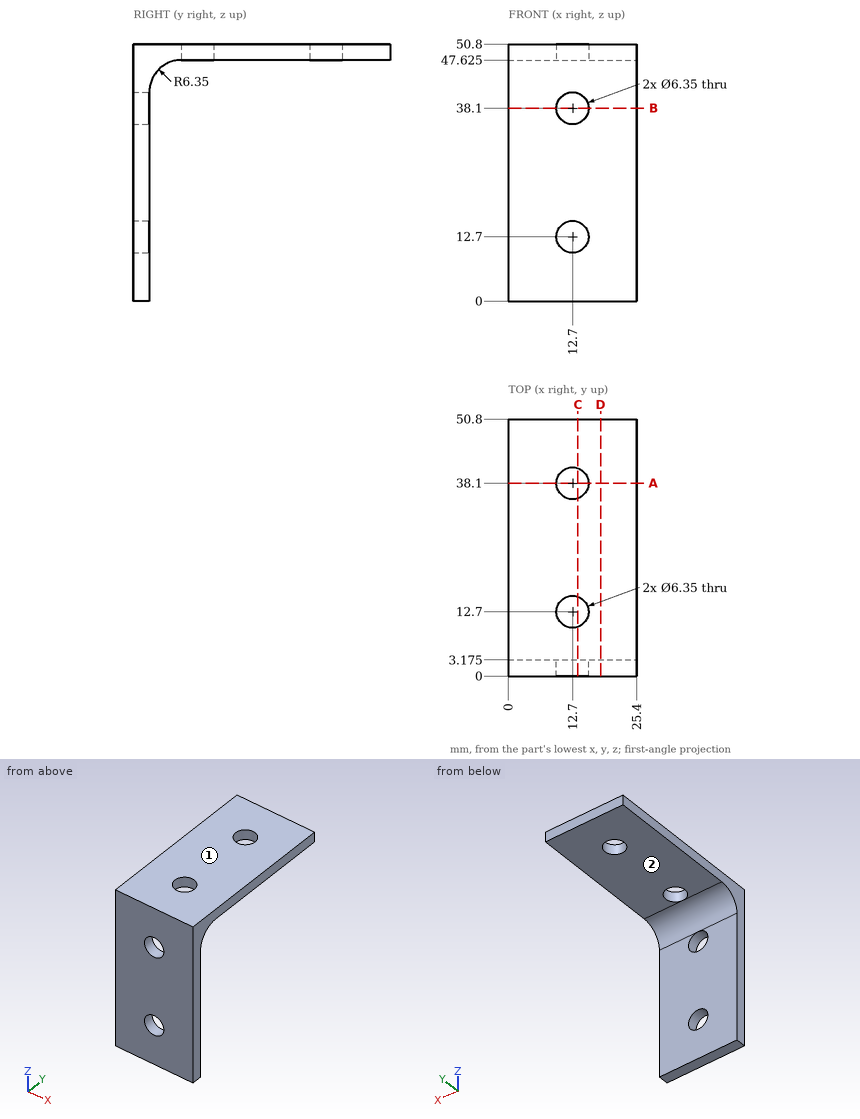
Study the drawing (mm; zero at the part's minimum x, y, z) and answer. A direction names the side the tool comes from. Give positions to 0.01 mm unless a question says otherwise; leave off trailing zeros. Order: outer loops, then holes, each group sorted by start corner. A loop starts at its lowest first (then second) coordinate and runs counter-clockwise, first axis right, second up.
1. Section A-A, the plane y = 38.1 is taken. Determine the outline of the cut face in (x, z) (3 decimals), and give its area (3 significant figures).
Result sheet:
outline: (0, 47.625) - (9.525, 47.625) - (9.525, 50.8) - (0, 50.8) - close; (15.875, 47.625) - (25.4, 47.625) - (25.4, 50.8) - (15.875, 50.8) - close
area: 60.5 mm2
2. For the marked faces 1 and 2, determine the directions among +Z, -Z, +X, -X, +Y, -Y from which every point of the face is accessible in a straight line to the end or side of a thin tool.
Result sheet:
face 1: +Z, +X, -X, +Y, -Y
face 2: -Z, +X, -X, +Y
3. Straight lines are drawn through the part: L1, parallel to Z at x = 12.7, y = 0.8 (3 decimals); L2, parallel to X at y = 38, z = 49. For each, find the intervals that lie inside material, in ascending order.
Result sheet:
L1: z = 0 to 9.525, 15.875 to 34.925, 41.275 to 50.8
L2: x = 0 to 9.53, 15.87 to 25.4
4. Section C-C, the plane x = 13.75 is taken. Determine the outline of the cut face in (y, z) (3 decimals), and give its area (3 significant figures).
Result sheet:
outline: (0, 0) - (3.175, 0) - (3.175, 9.704) - (0, 9.704) - close; (0, 15.696) - (3.175, 15.696) - (3.175, 35.104) - (0, 35.104) - close; (0, 41.096) - (3.175, 41.096) - (3.175, 41.275) arc R6.35 cw to (9.525, 47.625) - (9.704, 47.625) - (9.704, 50.8) - (0, 50.8) - close; (15.696, 47.625) - (35.104, 47.625) - (35.104, 50.8) - (15.696, 50.8) - close; (41.096, 47.625) - (50.8, 47.625) - (50.8, 50.8) - (41.096, 50.8) - close
area: 245 mm2
5. Each of these flat-tipped pins is pushed along its axis until it touches: P1, Ø8, axis at x = 22, y = 12, coming from the -Z side; P2, Ø4, axis at x = 12.7, y = 38.1, coming from the -Z side; P3, Ø1, axis at x = 15.5, z = 26.5, coming from the +Y side (3 decimals). Where does it stop, or does it pass through?
Result sheet:
P1: stops at z = 47.44
P2: passes through
P3: stops at y = 3.175
6. Section B-B, the plane z = 38.1 is taken. Determine the outline of the cut face in (x, y) (3 decimals), and give its area (3 significant figures).
Result sheet:
outline: (0, 0) - (9.525, 0) - (9.525, 3.175) - (0, 3.175) - close; (15.875, 0) - (25.4, 0) - (25.4, 3.175) - (15.875, 3.175) - close
area: 60.5 mm2
7. Section D-D, the plane x = 18.25 is taken. Determine the outline of the cut face in (y, z) (3 decimals), and give its area (3 significant figures).
Result sheet:
outline: (0, 0) - (3.175, 0) - (3.175, 41.275) arc R6.35 cw to (9.525, 47.625) - (50.8, 47.625) - (50.8, 50.8) - (0, 50.8) - close
area: 321 mm2
